Work out the finished part from the listing and answer in its coordinate system (mm). A direction names the side the tool comes from. Round coordinates to 2 decimals unless told otherwise and drop trailing zeros. Order: outer loops, then holes, each group sorted by start corner. A loop starts at its lowest first (then second) coordinate and runs counter-clockwise, first axis right, second up. Notation, with made-up numbers: (17.5, 70) - (60.5, 70) arc R28 ccw to (60.5, 89) - close; hole circle Ø10 at (20, 28). An arc over 180 degrees is marked (long way). One line per question, with ' | ' between items. Start each with the question number.
from build123d import *

# Parameters (mm, degrees)
SKETCH_W     = 89
SKETCH_H     = 25
PAD_DEPTH    = 42
SKETCH001_R  = 4
PAD001_DEPTH = 13
SKETCH002_W  = 31
SKETCH002_H  = 21
POCKET_DEPTH = 1


with BuildPart() as part:
    # Sketch → Pad (new body)
    with BuildSketch(Plane.XY):
        with Locations((44.5, -12.5)):
            Rectangle(SKETCH_W, SKETCH_H)
    extrude(amount=PAD_DEPTH)

    # Sketch001 (on Face5 of Pad) → Pad001 (join)
    with BuildSketch(Plane(origin=(0, 0, 0), x_dir=(1, 0, 0), z_dir=(0, 0, -1))):
        with Locations((85, 4)):
            Circle(SKETCH001_R)
        with Locations((4, 21)):
            Circle(SKETCH001_R)
    extrude(amount=PAD001_DEPTH)

    # Sketch002 (on Face6 of Pad001) → Pocket (cut)
    with BuildSketch(Plane.XY.offset(42)):
        with Locations((44.5, -12.5)):
            Rectangle(SKETCH002_W, SKETCH002_H)
    extrude(amount=-POCKET_DEPTH, mode=Mode.SUBTRACT)


solid = part.part
1) Straight lines are drawn through the part: line 1 (Z direction, x = 59.5, y = -5.5); line 2 (Z direction, x = 65, y = -4); line 3 (X direction, y = -24, z = -1). For each, find the intervals that lie inside material, in ascending order.
2) Section C-C on y = -12.25 is taken. Give the vertices of the cut face in (x, z), and give its area (3 significant figures).
3) Flat-ended cylindrical pins translate along their axes: pin 1 (3 mm diameter, centred on y = -22, z = -6.5, fed in from +X); pin 2 (6 mm diameter, centred on x = 23, y = -14.5, fed in from -Z); pin 3 (10.5 mm diameter, centred on x = 43, y = -11.5, fed in from +Z). Find the tip coordinate at first contact, or state that the pin passes through.
4) For faces 4 (the flat face through (1, -24, 0)), 5 (the flat face through (88, -1, 0)), 6 (the cylindrical face through (81, -4, -6)), determine the directions among +Z, -Z, +X, -X, +Y, -Y from which every point of the face is accessible in a straight line to the end or side of a thin tool.
5) Section A-A on x = 57 is taken. Give the vertices of the cut face in (y, z), and give its area (3 significant figures).
6) Section D-D on y = -20 is taken. Give the vertices of the cut face in (x, z).
7) Section B-B on z = -2 is taken. Give the vertices of the cut face in (x, y).
8) Determine the mould class of faces 1 (the flat face through (44, -12, 41)), 2 (the flat face through (0, -13, 21)), 3 (the flat face through (44, 0, 21)) for opening direction X: released by +X, released by -X, zero draft, split by the parting line, or undercut.
Recorded:
1) line 1: z = 0 to 41 | line 2: z = 0 to 42 | line 3: x = 1.35 to 6.65
2) outline: (0, 0) - (89, 0) - (89, 42) - (60, 42) - (60, 41) - (29, 41) - (29, 42) - (0, 42) - close | area: 3,710 mm²
3) pin 1: stops at x = 8 | pin 2: stops at z = 0 | pin 3: stops at z = 41
4) face 4: -Z, -X, -Y | face 5: -Z, +X, +Y | face 6: -Z
5) outline: (-25, 0) - (0, 0) - (0, 42) - (-2, 42) - (-2, 41) - (-23, 41) - (-23, 42) - (-25, 42) - close | area: 1,030 mm²
6) outline: (0, 0) - (0.13, 0) - (0.13, -13) - (7.87, -13) - (7.87, 0) - (89, 0) - (89, 42) - (60, 42) - (60, 41) - (29, 41) - (29, 42) - (0, 42) - close
7) outline: circle Ø8 at (4, -21); circle Ø8 at (85, -4)
8) face 1: undercut | face 2: released by -X | face 3: zero draft
